Design review of the part shown in the three views and the two pictorial views. Dimensions are in mm from the part's minimum x, y and z. A direction names the side the tool comes from. Coordinates: 2 decimals unless noted, no trailing zeros. Loops run counter-clockwise (first coordinate to the right, second up) from the corner with the lowest first, then second, coordinate; pieces in that order, holes last. Notation, with made-up numbers: M 52,21 L 104,21 A30 cw 104,59 Z; hole C -32.5,-30 d1. An arc over 180 degrees is marked long. Put each result on its own line as item: value. Start each with the question number.
(1) Clearance check with flat-ended pins moving along their axes: pin 1 (6.5 mm diameter, centred on y = 45, z = 26.5, fed in from -X); pin 2 (4 mm diameter, centred on x = 43.5, y = 41.5, fed in from -Z); pin 3 (12 mm diameter, centred on x = 38.5, y = 31, fed in from +Z). State where each tip first meets the part, or that it passes through.
(2) Take a section at B-B, the plane z = 65.5. Give the boundary of the cut face in (x, y), then the cut area to 3 significant figures.
(3) Take a section at C-C, the plane z = 26.5. Give the boundary of the cut face in (x, y), then the cut area to 3 significant figures.
(4) For probe 1 along Y at (x, z) = (68, 26.5); probe 2 along Y at (x, z) = (21.5, 1); probe 3 along X at (y, z) = (33, 69), list the stretches that pass through material, from the lowest coordinate up. Write a range as [from, to].
(5) Take a section at D-D, the plane x = 46.5. Give the boundary of the cut face in (y, z).
(6) Take a section at A-A, the plane x = 7.5. Give the boundary of the cut face in (y, z).
(7) For the marked faces 1 and 2, list the 3-axis set-ups (+Z, -Z, +X, -X, +Y, -Y) from which the entire face can be reached by the end or side of a thin tool; tool diameter is ignored.
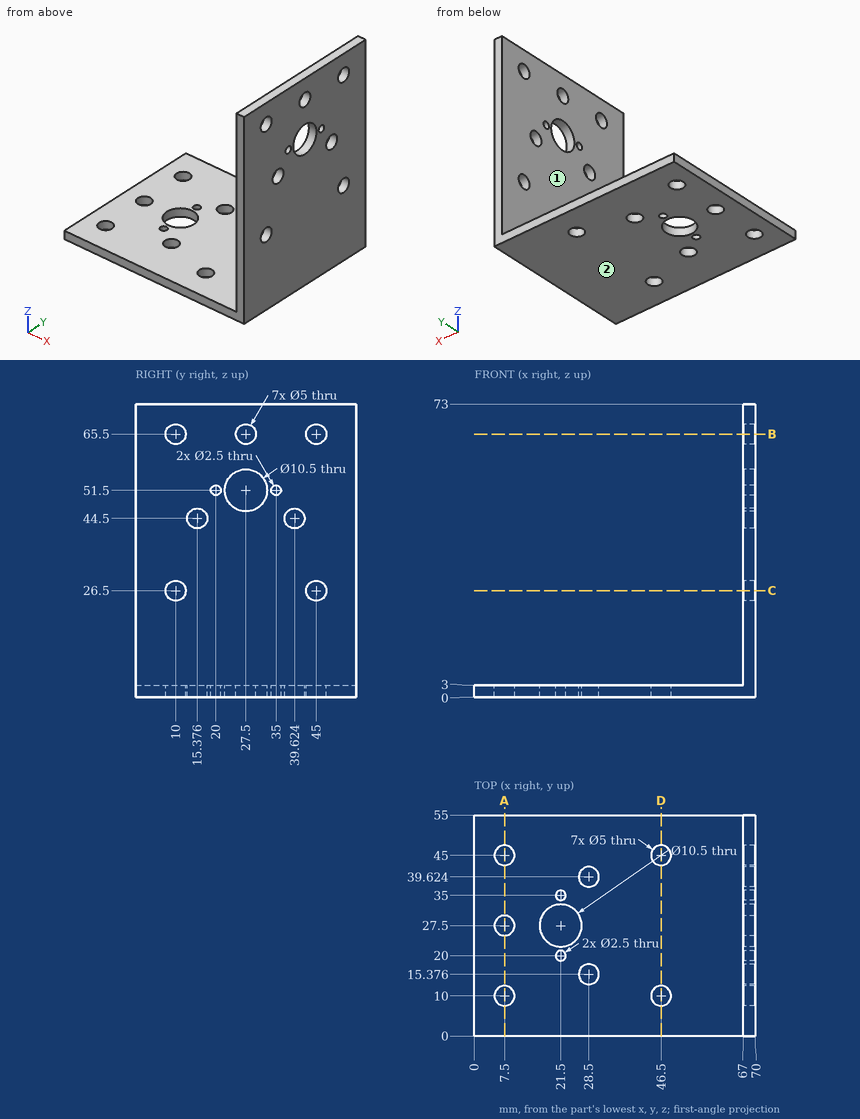
Computed values:
1. pin 1: stops at x = 67
1. pin 2: stops at z = 0
1. pin 3: stops at z = 3
2. outline: M 67,0 L 70,0 L 70,7.5 L 67,7.5 Z; M 67,12.5 L 70,12.5 L 70,25 L 67,25 Z; M 67,30 L 70,30 L 70,42.5 L 67,42.5 Z; M 67,47.5 L 70,47.5 L 70,55 L 67,55 Z
2. area: 120 mm^2
3. outline: M 67,0 L 70,0 L 70,7.5 L 67,7.5 Z; M 67,12.5 L 70,12.5 L 70,42.5 L 67,42.5 Z; M 67,47.5 L 70,47.5 L 70,55 L 67,55 Z
3. area: 135 mm^2
4. probe 1: y = [0, 7.5], [12.5, 42.5], [47.5, 55]
4. probe 2: y = [0, 18.75], [21.25, 22.25], [32.75, 33.75], [36.25, 55]
4. probe 3: x = [67, 70]
5. outline: M 0,0 L 7.5,0 L 7.5,3 L 0,3 Z; M 12.5,0 L 42.5,0 L 42.5,3 L 12.5,3 Z; M 47.5,0 L 55,0 L 55,3 L 47.5,3 Z
6. outline: M 0,0 L 7.5,0 L 7.5,3 L 0,3 Z; M 12.5,0 L 25,0 L 25,3 L 12.5,3 Z; M 30,0 L 42.5,0 L 42.5,3 L 30,3 Z; M 47.5,0 L 55,0 L 55,3 L 47.5,3 Z
7. face 1: +Z, -X, +Y, -Y
7. face 2: -Z, +X, -X, +Y, -Y
